Could you check a few things on this drawing? It's one solid part, dimensions in mm from its lowest x, y, z. A direction names the side the tool comes from. Coordinates: 2 decimals unless noted, no trailing zeros. Loops run counter-clockwise (first coordinate to the right, second up) from the corner with the lowest first, then second, coordinate; pieces in that order, holes last. Notation, with made-up numbers: M -24,9 L 5,9 A17 cw 5,22 Z; hole C 35,-36.5 d2. An arc over 180 degrees is marked long. Use one line per item in the form item = value. Start each with the question number.
(1) On a 3-axis mill with a long thin cutter (end or side, diameter ignored), from which of +Z, -Z, +X, -X, +Y, -Y can I reach the whole of each face in a straight line? I mean the marked faces 4 and 5. Say none if no direction works.
(2) Imagine slicing it at C-C, the plane z = 34. Please give me the cut outline in (x, y) (1 decimal).
(3) Will these pins go through, and if not, where does the flat tip stop? P1, Ø16.5, axis at x = 19.05, y = 19.05, coming from the +Z side; P2, Ø5, axis at y = 20, z = 25.5, coming from the +X side; P3, Ø15, axis at x = 63.5, z = 25.4, coming from the -Y side (3 decimals).
(4) Imagine slicing it at B-B, the plane x = 19.05. Please give me the cut outline in (y, z).
(5) Imagine slicing it at A-A, the plane y = 19.05. State how many separate pieces and enclosed holes the cut face has, and give its area (3 significant figures).
(6) Thinking about a two-plate mould opening in Z: for the marked faces 1, 2 and 3, which applies, +Z half, -Z half, draft (parallel to the pull), parting line (faces both ways), or undercut?
(7) Please list where these lines run through material, in increasing order: L1, parallel to Z at x = 63, y = 20; L2, parallel to Y at x = 107.95, z = 9.75; L3, parallel to X at y = 24.5, z = 2.5 (1 decimal).
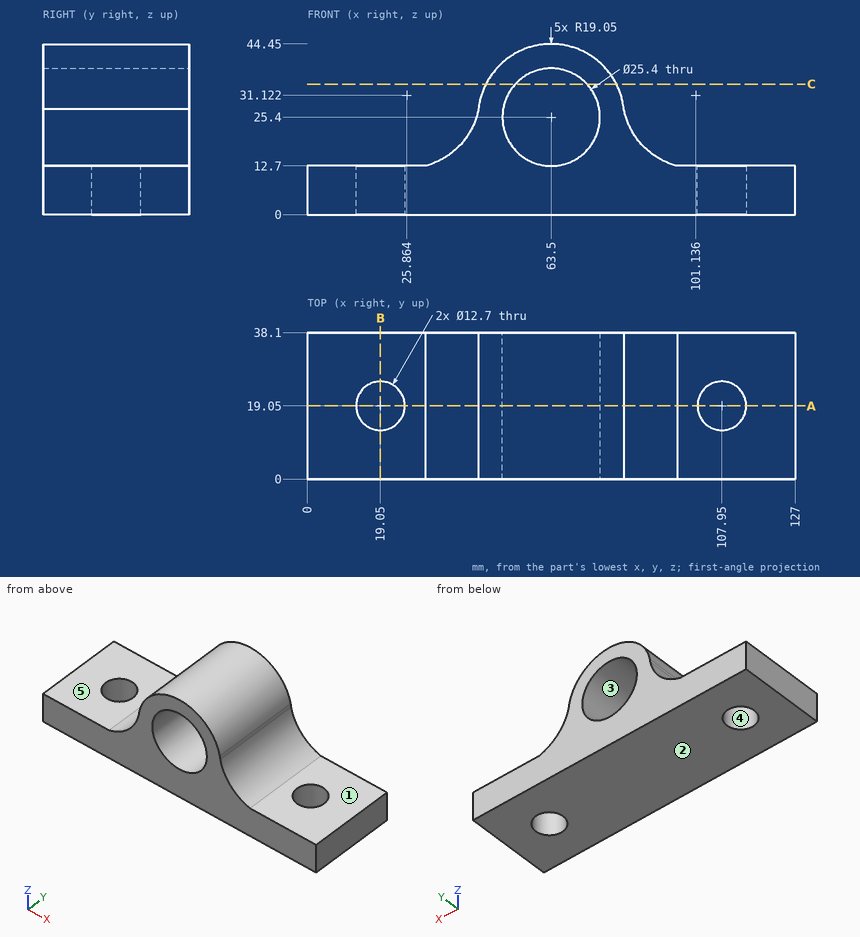
Answer:
q1.face_4 = +Z, -Z
q1.face_5 = +Z, -X, +Y, -Y
q2.outline = M 46.5,0 L 54.2,0 L 54.2,38.1 L 46.5,38.1 Z; M 72.8,0 L 80.5,0 L 80.5,38.1 L 72.8,38.1 Z
q3.P1 = 12.7
q3.P2 = 83.9
q3.P3 = through
q4.outline = M 0,0 L 12.7,0 L 12.7,12.7 L 0,12.7 Z; M 25.4,0 L 38.1,0 L 38.1,12.7 L 25.4,12.7 Z
q5.separate_pieces = 3
q5.enclosed_holes = 1
q5.area = 1,960 mm²
q6.face_1 = +Z half
q6.face_2 = -Z half
q6.face_3 = undercut
q7.L1 = 0 to 12.71, 38.09 to 44.44
q7.L2 = 0 to 12.7, 25.4 to 38.1
q7.L3 = 0 to 15.8, 22.3 to 104.7, 111.2 to 127
